Here's how the part is built. I have some questions about the finished solid (model axes, mm). Face numbers are marked on the shaded views. A direction names the side the tool comes from. Round coordinates to 2 decimals unless told otherwise and drop trailing zeros. Loops run counter-clockwise (first coordinate to the right, second up) from the corner with the lowest first, then second, coordinate; pieces in that order, holes last. Notation, with made-up numbers: M 77,51.5 L 98,51.5 A30 ccw 98,75.5 Z; hole C 68.5,3 d11. An arc over 180 degrees is marked long. Answer as CSV lines item,"result".
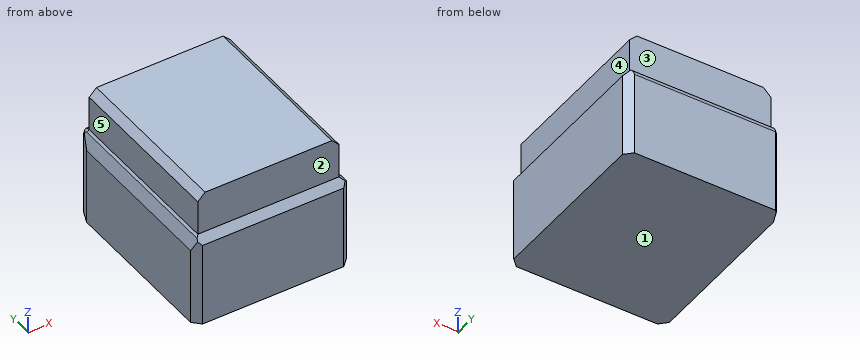
```python
from build123d import *

# Parameters (mm, degrees)
F0_W         = 109.1705858707
F0_H         = 127.4348646402
F1_DEPTH     = 64.262
F2_SIZE      = 5.08
F3_R         = 5.08
F4_SIZE      = 5.08
F5_SIZE      = 5.08
F6_T1_DEPTH  = 85.5235311919
F7_SIZE      = 5.08
F8_SIZE      = 5.08
F9_SIZE      = 5.08
F10_DEPTH    = 29.464
F11_T1_DEPTH = 138.5363958322
F11_T3_DEPTH = 143.403163798


# Not quite as in the source:
# - a fillet or chamfer that OpenCascade refuses, or shapes differently, is made with other operations: its cross-section is extruded or revolved along the edge and cut away or added
# - two fillets or chamfers of one size are made in one step


with BuildPart() as f1:
    # F0 (on Top) → F1 (new body)
    with BuildSketch(Plane.XY):
        with Locations((2.4905838072, 0.1037716866)):
            Rectangle(F0_W, F0_H)
    extrude(amount=F1_DEPTH)

    # F2
    f2_edges = [f1.edges().sort_by_distance(p)[0] for p in [
        (57.075877, 0.103772, 64.262),
    ]]
    chamfer(f2_edges, length=F2_SIZE)

    # F3
    f3_edges = [f1.edges().sort_by_distance(p)[0] for p in [
        (-0.049416, 63.821204, 64.262),
    ]]
    fillet(f3_edges, radius=F3_R)

    # F4
    f4_edges = [f1.edges().sort_by_distance(p)[0] for p in [
        (-0.049416, -63.613661, 64.262),
    ]]
    chamfer(f4_edges, length=F4_SIZE)

    # F5
    f5_edges = [f1.edges().sort_by_distance(p)[0] for p in [
        (-52.094709, 0.103772, 64.262),
    ]]
    chamfer(f5_edges, length=F5_SIZE)

    # F6: chamfer of 5.08 on 1 edges, made by hand

    # F6_s2 → F6_t1 (cut)
    with BuildSketch(Plane.XY.offset(-13.170765596)):
        Polygon((-52.0947091281, 53.6612040067), (-48.5026066797, 62.3333064551), (-52.0947091281, 58.7412040067), align=None)
    extrude(amount=F6_T1_DEPTH, mode=Mode.SUBTRACT)

    # F7
    f7_edges = [f1.edges().sort_by_distance(p)[0] for p in [
        (-52.094709, -63.613661, 29.591),
    ]]
    chamfer(f7_edges, length=F7_SIZE)

    # F8
    f8_edges = [f1.edges().sort_by_distance(p)[0] for p in [
        (57.075877, -63.613661, 29.591),
    ]]
    chamfer(f8_edges, length=F8_SIZE)

    # F9
    f9_edges = [f1.edges().sort_by_distance(p)[0] for p in [
        (57.075877, 63.821204, 29.591),
    ]]
    chamfer(f9_edges, length=F9_SIZE)

    # F10 (add): a face of the model
    f10_faces = [f1.faces().sort_by_distance(p)[0] for p in [
        (2.4905838072, 0.1037716866, 64.262),
    ]]
    extrude(f10_faces, amount=F10_DEPTH)

    # F11: chamfer of 5.08 on 3 edges, made by hand

    # F11_s2 → F11_t1 (cut)
    with BuildSketch(Plane.XZ.offset(-66.8319696027)):
        Polygon((-52.0947091281, 54.102), (-48.5026066797, 62.7741024484), (-52.0947091281, 59.182), align=None)
    extrude(amount=F11_T1_DEPTH, mode=Mode.SUBTRACT)

    # F11_s4 → F11_t3 (cut)
    with BuildSketch(Plane.XZ.offset(-71.8053535855)):
        Polygon((51.9958767426, 88.646), (46.9158767426, 93.726), (51.9958767426, 93.726), align=None)
        Polygon((-47.0147091281, 88.646), (-41.9347091281, 93.726), (-47.0147091281, 93.726), align=None)
    extrude(amount=F11_T3_DEPTH, mode=Mode.SUBTRACT)


solid = f1.part
```
1. If I drill on line 1 (Y direction, x = 29.5, z = 86.5); line 2 (X direction, y = 18, z = 77); line 3 (X direction, y = -28.5, z = 58.5), over which ranges is the centre line in solid material (lowest first)? Write a range as [from, to].
Evaluation:
line 1,"y = [-58.53, 58.74]"
line 2,"x = [-47.01, 52]"
line 3,"x = [-50.27, 57.08]"
2. I want a section at A-A, the plane x = -32. Please give me the cut outline in (y, z), and give its area (3 significant figures).
Evaluation:
outline,"M -63.61,0 L 63.82,0 L 63.82,59.18 A5.08 ccw 58.74,64.26 L 58.74,93.73 L -58.53,93.73 L -58.53,64.26 L -63.61,59.18 Z"
area,"11,600 mm²"
3. I want a section at B-B, the plane y = 7.5. Please give me the cut outline in (x, z), and give its area (3 significant figures).
Evaluation:
outline,"M -52.09,0 L 57.08,0 L 57.08,59.18 L 52,64.26 L 52,88.65 L 46.92,93.73 L -41.93,93.73 L -47.01,88.65 L -47.01,64.26 L -48.5,62.77 L -52.09,54.1 Z"
area,"9,870 mm²"
4. For P1, Ø19.5, axis at y = -10, z = 71.5, coming from the +X side; P2, Ø14.5, axis at x = -2, z = 80, coming from the +Y side; P3, Ø7.5, axis at y = -10, z = 77.5, coming from the -X side, each with a flat end and sliding along its axis, tell me the tip position at first contact or that it passes through.
Evaluation:
P1,"stops at x = 54.51"
P2,"stops at y = 58.74"
P3,"stops at x = -47.01"
5. Which directions (+Z, -Z, +X, -X, +Y, -Y) give clear straight access to the entire face, cutting with the end or side of a thin tool? Please do the marked faces 1, 2, 3, 4 and 5.
Evaluation:
face 1,"-Z, +X, -X, +Y, -Y"
face 2,"+Z, +X, -X, -Y"
face 3,"+Z, +X, -X, +Y"
face 4,"+Z, +X, +Y, -Y"
face 5,"+Z, -X, +Y, -Y"
